Part model, mm, in its own coordinate system. Give positions to 0.01 mm unless a question says otherwise; leave off trailing zeros. Write each loop counter-clockwise with the first axis right and the second up, starting at its lowest first coordinate (ties: lowest second). Pieces come first, ordered by that corner, then holes. Notation, with made-up numbers: (55, -34.5) - (75, -34.5) arc R26 cw to (75, 1.5) - close; hole circle Ø8 at (57.25, 71). An arc over 180 degrees is marked (long way). Answer as a JSON object with one key per item and string values. Group by question number.
```python
from build123d import *

# Parameters (mm, degrees)
SCHIZZO1_W                   = 558
SCHIZZO1_H                   = 438
ESTRUSIONE_ESTRUSIONE1_DEPTH = 6
SCHIZZO2_R                   = 2.25
TAGLIO_ESTRUSIONE1_DEPTH     = 10
SCHIZZO4_R                   = 3.3
TAGLIO_ESTRUSIONE2_DEPTH     = 10
SCHIZZO5_R                   = 2.25
TAGLIO_ESTRUSIONE3_DEPTH     = 10
TAGLIO_ESTRUSIONE4_DEPTH     = 10


with BuildPart() as part:
    # Schizzo1 → Estrusione-Estrusione1 (new body)
    with BuildSketch(Plane(origin=(0, 0, 0), x_dir=(1, 0, 0), z_dir=(0, 1, 0))):
        Rectangle(SCHIZZO1_W, SCHIZZO1_H)
    extrude(amount=ESTRUSIONE_ESTRUSIONE1_DEPTH)

    # Schizzo2 → Taglio-Estrusione1 (cut)
    with BuildSketch(Plane(origin=(0, 6, 0), x_dir=(1, 0, 0), z_dir=(0, 1, 0))):
        with Locations(Location((-231, 205.5, 0), (0, 0, 270))):
            Circle(SCHIZZO2_R)
        with Locations(Location((-231, 187, 0), (0, 0, 270))):
            Circle(SCHIZZO2_R)
        with Locations(Location((-247, 171, 0), (0, 0, 270))):
            Circle(SCHIZZO2_R)
        with Locations(Location((-265.5, 171, 0), (0, 0, 270))):
            Circle(SCHIZZO2_R)
        with Locations(Location((231, 205.5, 0), (0, 0, 270))):
            Circle(SCHIZZO2_R)
        with Locations(Location((231, 187, 0), (0, 0, 270))):
            Circle(SCHIZZO2_R)
        with Locations(Location((247, 171, 0), (0, 0, 270))):
            Circle(SCHIZZO2_R)
        with Locations(Location((265.5, 171, 0), (0, 0, 270))):
            Circle(SCHIZZO2_R)
        with Locations(Location((265.5, -171, 0), (0, 0, 270))):
            Circle(SCHIZZO2_R)
        with Locations(Location((247, -171, 0), (0, 0, 270))):
            Circle(SCHIZZO2_R)
        with Locations(Location((231, -187, 0), (0, 0, 270))):
            Circle(SCHIZZO2_R)
        with Locations(Location((231, -205.5, 0), (0, 0, 270))):
            Circle(SCHIZZO2_R)
        with Locations(Location((-231, -205.5, 0), (0, 0, 270))):
            Circle(SCHIZZO2_R)
        with Locations(Location((-231, -187, 0), (0, 0, 270))):
            Circle(SCHIZZO2_R)
        with Locations(Location((-247, -171, 0), (0, 0, 270))):
            Circle(SCHIZZO2_R)
        with Locations(Location((-265.5, -171, 0), (0, 0, 270))):
            Circle(SCHIZZO2_R)
    extrude(amount=-TAGLIO_ESTRUSIONE1_DEPTH, mode=Mode.SUBTRACT)

    # Schizzo4 → Taglio-Estrusione2 (cut)
    with BuildSketch(Plane(origin=(0, 6, 0), x_dir=(1, 0, 0), z_dir=(0, 1, 0))):
        with Locations(Location((-11.04713937, -29.950902322, 0), (0, 0, 270))):
            Circle(SCHIZZO4_R)
        with Locations(Location((97.170402481, -88.545989873, 0), (0, 0, 270))):
            Circle(SCHIZZO4_R)
        with Locations(Location((155.765489817, 19.671552094, 0), (0, 0, 270))):
            Circle(SCHIZZO4_R)
        with Locations(Location((47.547947967, 78.266639645, 0), (0, 0, 270))):
            Circle(SCHIZZO4_R)
    extrude(amount=-TAGLIO_ESTRUSIONE2_DEPTH, mode=Mode.SUBTRACT)

    # Schizzo5 → Taglio-Estrusione3 (cut)
    with BuildSketch(Plane.XZ):
        with Locations(Location((-136.921607377, 165.135242981, 0), (0, 0, 270))):
            Circle(SCHIZZO5_R)
        with Locations(Location((-136.921607377, 145.135242981, 0), (0, 0, 270))):
            Circle(SCHIZZO5_R)
    extrude(amount=-TAGLIO_ESTRUSIONE3_DEPTH, mode=Mode.SUBTRACT)

    # Schizzo6 → Taglio-Estrusione4 (cut)
    with BuildSketch(Plane(origin=(0, 6, 0), x_dir=(1, 0, 0), z_dir=(0, 1, 0))):
        Polygon((-279, 0), (-261.3, 0), (-268.8, 10), (-233.4, 10), (-240.9, 0), (-223.2, 0), (-205.5, 0), (-213, 10), (-177.6, 10), (-185.1, 0), (-167.4, 0), (-149.7, 0), (-157.2, 10), (-121.8, 10), (-129.3, 0), (-111.6, 0), (-93.9, 0), (-101.4, 10), (-66, 10), (-73.5, 0), (-55.8, 0), (-38.1, 0), (-45.6, 10), (-10.2, 10), (-17.7, 0), (0, 0), (17.7, 0), (10.2, 10), (45.6, 10), (38.1, 0), (55.8, 0), (73.5, 0), (66, 10), (101.4, 10), (93.9, 0), (111.6, 0), (129.3, 0), (121.8, 10), (157.2, 10), (149.7, 0), (167.4, 0), (185.1, 0), (177.6, 10), (213, 10), (205.5, 0), (223.2, 0), (240.9, 0), (233.4, 10), (268.8, 10), (261.3, 0), (279, 0), (279, -219), (-279, -219), align=None)
    extrude(amount=-TAGLIO_ESTRUSIONE4_DEPTH, mode=Mode.SUBTRACT)


solid = part.part
```
1) Drop flat-ended pins along their axis: P1, Ø1.8, axis at x = 75.5, y = 1.5, coming from the +Z side; P2, Ø4, axis at x = 63.5, z = -114, coming from the -Y side. Give the stop position or say it passes through.
2) Band-saw the part on B-B (y = 3.7). State how many separate pieces and enclosed holes the cut face has, plus the area to 3 significant figures.
3) Band-saw the part on A-A (x = 193.5). List the corners of the cut face in (y, z), plus the area to 3 significant figures.
4) Probe line 1 (X direction, y = 4.75, z = -205.5); line 2 (X direction, y = 2.6, z = -171); line 3 (Z direction, x = 231, y = 4.1). List the from-to ranges inside material, lowest first.
Verdict:
{
 "1": {"P1": "z = -10", "P2": "y = 0"},
 "2": {"separate pieces": "1", "enclosed holes": "10", "area": "119,000 mm2"},
 "3": {"outline": "(0, -219) - (6, -219) - (6, -10) - (0, -10) - close", "area": "1,250 mm2"},
 "4": {"line 1": "-279 to -233.25, -228.75 to 228.75, 233.25 to 279", "line 2": "-279 to -267.75, -263.25 to -249.25, -244.75 to 244.75, 249.25 to 263.25, 267.75 to 279", "line 3": "-219 to -207.75, -203.25 to -189.25, -184.75 to 0"}
}
